from build123d import *

# Parameters (mm, degrees)
F0_R      = 90
F1_DEPTH  = 5
F2_R      = 67.5
F3_DEPTH  = 5
F4_R      = 2.5
F5_DEPTH  = 5.001
F7_DEPTH  = 5.001
F9_DEPTH  = 2.5
F11_DEPTH = 2.501
F13_DEPTH = 2.501
F15_DEPTH = 2.501
F19_DEPTH = 2.5


with BuildPart() as f1:
    # F0 (on Top) → F1 (new body)
    with BuildSketch(Plane.XY):
        Circle(F0_R)
    extrude(amount=F1_DEPTH)

    # F2 (on face) → F3 (cut)
    with BuildSketch(Plane.XY.offset(5)):
        Circle(F2_R)
    extrude(amount=-F3_DEPTH, mode=Mode.SUBTRACT)

    # F4 (on face) → F5 (cut, through all)
    with BuildSketch(Plane.XY.offset(5)):
        with Locations((0, 80)):
            Circle(F4_R)
    extrude(amount=-F5_DEPTH, mode=Mode.SUBTRACT)

    # F6 (on face) → F7 (cut, through all)
    with BuildSketch(Plane.XY.offset(5)):
        with BuildLine():
            ThreePointArc((49.1439212925, 49.1439212925), (51.8683968263, 48.6019894142), (53.4116882454, 50.9116882454))
            ThreePointArc((53.4116882454, 50.9116882454), (49.9549796645, 53.2213870767), (49.1439212925, 49.1439212925))
        make_face()
    extrude(amount=-F7_DEPTH, mode=Mode.SUBTRACT)

    # F8 (on face) → F9 (cut)
    with BuildSketch(Plane.XY.offset(5)):
        with BuildLine():
            Line((-28.5267326675, 61.175775625), (-38.0356435567, 81.5677008333))
            ThreePointArc((-38.0356435567, 81.5677008333), (-30.7818128993, -84.5723358707), (81.5677008333, 38.0356435567))
            Line((81.5677008333, 38.0356435567), (61.175775625, 28.5267326675))
            ThreePointArc((61.175775625, 28.5267326675), (-23.0863596745, -63.429251903), (-28.5267326675, 61.175775625))
        make_face()
    extrude(amount=-F9_DEPTH, mode=Mode.SUBTRACT)

    # F10 (on face) → F11 (cut, through all)
    with BuildSketch(Plane.XY.offset(2.5)):
        with BuildLine():
            ThreePointArc((77.0361638276, 35.9225531477), (-29.0717129108, -79.8738747674), (-35.9225531477, 77.0361638276))
            Line((-35.9225531477, 77.0361638276), (-38.0356435567, 81.5677008333))
            ThreePointArc((-38.0356435567, 81.5677008333), (-48.3569647512, -75.9052301232), (90, 0))
            ThreePointArc((90, 0), (87.8666406408, 19.4795652544), (81.5677008333, 38.0356435567))
            Line((81.5677008333, 38.0356435567), (77.0361638276, 35.9225531477))
        make_face()
    extrude(amount=-F11_DEPTH, mode=Mode.SUBTRACT)

    # F12 (on face) → F13 (cut, through all)
    with BuildSketch(Plane.XY.offset(2.5)):
        with BuildLine():
            Line((-28.5267326675, 61.175775625), (-30.6398239762, 65.7073145602))
            ThreePointArc((-30.6398239762, 65.7073145602), (-24.7964603911, -68.127715007), (65.7073145602, 30.6398239762))
            Line((65.7073145602, 30.6398239762), (61.175775625, 28.5267326675))
            ThreePointArc((61.175775625, 28.5267326675), (65.8999804806, 14.6096739408), (67.5, 0))
            ThreePointArc((67.5, 0), (-36.2677235634, -56.9289225924), (-28.5267326675, 61.175775625))
        make_face()
    extrude(amount=-F13_DEPTH, mode=Mode.SUBTRACT)

    # F14 (on face) → F15 (cut, through all)
    with BuildSketch(Plane.XY.offset(2.5)):
        Polygon((98.6606093618, 26.4360306033), (0, 0), (-50.3402867184, 107.9550932479), (-138.5994553566, -33.6444936693), (-65.9655109048, -85.6016203761), (32.1168266237, -89.8430198431), (88.8455361128, -67.5756856799), align=None)
    extrude(amount=-F15_DEPTH, mode=Mode.SUBTRACT)

    # F18 (on face) → F19 (cut)
    with BuildSketch(Plane(origin=(0, 0, 0), x_dir=(1, 0, 0), z_dir=(0, 0, -1))):
        with BuildLine():
            Line((-21.9996188337, -82.1036952346), (-18.7643804985, -70.029621393))
            ThreePointArc((-18.7643804985, -70.029621393), (-24.7964600325, -68.1277140216), (-30.639823533, -65.7073136098))
            Line((-30.639823533, -65.7073136098), (-35.922552248, -77.0361618981))
            ThreePointArc((-35.922552248, -77.0361618981), (-29.0717121827, -79.8738727668), (-21.9996188337, -82.1036952346))
        make_face()
    extrude(amount=-F19_DEPTH, mode=Mode.SUBTRACT)


solid = f1.part
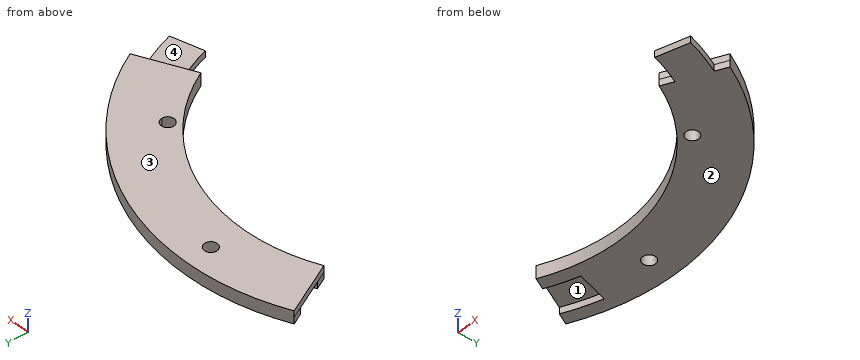
Geometry: final body of the model. Coordinates: model frame, mm. Face numbers are marked on the shaded views. A direction names the side the tool comes from. Coordinates: 2 decimals unless noted, no trailing zeros. Order: outer loops, then holes, each group sorted by start corner. A loop starts at its lowest first (then second) coordinate and runs counter-clockwise, first axis right, second up.
(1) First-contact query: pin 1 (3 mm diameter, centred on x = 64, z = 3.5, fed in from +Y); pin 2 (1.5 mm diameter, centred on y = 39.5, z = 2.5, fed in from -X); pin 3 (5 mm diameter, centred on x = 73, y = 23.5, fed in from +Z). Flat tips, straight axial feed; report the tip coordinate or a pass-through.
(2) Section query B-B (z = 4.2). Return the cut outline in (x, y), plus the area to 3 significant figures.
(3) Access query for the marked faces 3 and 4. Directions: +Z, -Z, +X, -X, +Y, -Y. A direction counts if a zero-diameter tool reaches every point of the face in a straight line with its end or side. Return the directions, or none.
(4) Section query D-D (x = -25). Return the cut outline in (y, z).
(5) Section query A-A (x = 0). Return the cut outline in (y, z).
(6) Material intervals for probe 1 along Y at (x, z) = (67.5, 4.65); probe 2 along Y at (x, z) = (15.5, 2.35); probe 3 along X at (y, z) = (47, 0.4), sorted ascending.
(7) Draft query along X for the marked faces 1 and 2. Return one class per face: pulls with the +X half, pulls with the -X half, needs draft (parallel to the pull), parting line crosses it, or undercut.
(8) Section query C-C (y = 80). Return the cut outline in (x, z).
Solution:
1. pin 1: stops at y = 64.76
1. pin 2: stops at x = 54.19
1. pin 3: stops at z = 2.5
2. outline: (-38.04, 81.57) - (-28.53, 61.18) arc R67.5 cw to (61.18, 28.53) - (81.57, 38.04) arc R90 ccw to start; hole circle Ø5 at (0, 80); hole circle Ø5 at (50.91, 50.91)
2. area: 2,740 mm2
3. face 3: +Z, +X, -X, +Y, -Y
3. face 4: +Z, +X, -Y
4. outline: (62.7, 0) - (68.05, 0) - (68.05, 2.5) - (81.24, 2.5) - (81.24, 0) - (86.46, 0) - (86.46, 5) - (62.7, 5) - close
5. outline: (67.5, 0) - (77.5, 0) - (77.5, 5) - (67.5, 5) - close; (82.5, 0) - (90, 0) - (90, 5) - (82.5, 5) - close
6. probe 1: y = 31.48 to 59.53
6. probe 2: y = 65.7 to 88.66
6. probe 3: x = 48.45 to 76.75
7. face 1: undercut
7. face 2: needs draft
8. outline: (-37.3, 0) - (-28.72, 0) - (-28.72, 2.5) - (-21.44, 2.5) - (-21.44, 0) - (-2.5, 0) - (-2.5, 5) - (-37.3, 5) - close; (2.5, 0) - (41.23, 0) - (41.23, 5) - (2.5, 5) - close
